Read the model definition and answer for the solid it produces. Units are mm, in the model's axes. Coordinates: 2 decimals unless noted, no trailing zeros. Order: outer loops, then holes, each group sorted by start corner. A loop starts at its lowest first (then second) coordinate and runs counter-clockwise, first axis right, second up. Notation, with made-up numbers: M 55,73.5 L 60,73.5 A14 cw 60,97.5 Z; hole C -32,27.5 d5. An arc over 180 degrees is marked long. Write each question's results on one line, items separated by ' | '.
Autodesk Inventor part; units mm, degrees
ref_plane "YZ Plane" through (0, 0, 0) normal (1, 0, 0) x (0, 1, 0)
ref_plane "XZ Plane" through (0, 0, 0) normal (0, 1, 0) x (-1, 0, 0)
ref_plane "XY Plane" through (0, 0, 0) normal (0, 0, 1) x (1, 0, 0)
sketch "Sketch1" plane through (0, 0, 0) normal (0, 1, 0) x (-1, 0, 0)
  line L0 (0, 0) -> (-95, 0)
  line L1 (-95, 0) -> (-95, -95)
  line L2 (-95, -95) -> (0, -95)
  line L3 (0, -95) -> (0, 0)
  line L4 (0, 0) -> (-5, 0)
  line L5 (-5, 0) -> (-5, -5)
  line L6 (-5, -5) -> (0, -5)
  line L7 (0, -5) -> (0, 0)
  line L8 (-95, -95) -> (-90, -95)
  line L9 (-90, -95) -> (-90, -90)
  line L10 (-90, -90) -> (-95, -90)
  line L11 (-95, -90) -> (-95, -95)
  line L12 (-90, -90) -> (-5, -90)
  line L13 (-5, -90) -> (-5, -5)
  line L14 (-5, -5) -> (-90, -5)
  line L15 (-90, -5) -> (-90, -90)
  line L16 (0, -47.5) -> (0, 0)
  line L17 (0, -47.5) -> (0, -95)
  line L18 (0, -23.75) -> (0, -18.75)
  line L19 (0, -18.75) -> (0, -28.75)
  line L20 (0, -71.25) -> (0, -76.25)
  line L21 (0, -76.25) -> (0, -66.25)
  line L22 (0, -18.75) -> (0, -28.75) construction
  line L23 (-5, -18.75) -> (-5, -28.75)
  line L24 (5, -28.75) -> (5, -18.75)
  arc A0 (5, -18.75) -> (-5, -18.75) centre (0, -18.75) ccw
  arc A1 (-5, -28.75) -> (5, -28.75) centre (0, -28.75) ccw
  line L25 (0, -66.25) -> (0, -76.25) construction
  line L26 (-5, -66.25) -> (-5, -76.25)
  line L27 (5, -76.25) -> (5, -66.25)
  arc A2 (5, -66.25) -> (-5, -66.25) centre (0, -66.25) ccw
  arc A3 (-5, -76.25) -> (5, -76.25) centre (0, -76.25) ccw
  point P0 (0, -61.25)
  point P1 (0, -81.25)
  point P2 (0, -13.75)
  point P3 (0, -33.75)
  dimension "d0" = 95
  dimension "d1" = 95
  dimension "d2" = 5
  dimension "d3" = 5
  dimension "d4" = 5
  dimension "d5" = 5
  dimension "d8" = 5
  dimension "d9" = 10
  dimension "d10" = 5
  dimension "d11" = 10
  dimension "d12" = 10
  dimension "d13" = 10
extrude "Extrusion1" add sketch "Sketch1" along normal blind 1.5 contours L3 L6 L5 L0 | L5 L14 L15 L10 L1 L0 | L3 A0 L13 L6 | A0 L24 A1 L3 | L3 A1 L13 A0 | L10 L9 L2 L1 | L12 L13 A3 L3 L2 L9 | A1 L3 A2 L13 | A2 L3 A3 L13 | A2 L27 A3 L3
fillet "Fillet1" radius 8 8 edges at (5, 0.75, -5) (0, 0.75, 0) (0, 0.75, -95) (5, 0.75, -90) (95, 0.75, 0) (90, 0.75, -5) (95, 0.75, -95) (90, 0.75, -90)
fillet "Fillet2" radius 1 12 edges at (-3.5355, 0, -15.2145) (-3.5355, 0, -32.2855) (-5, 0, -23.75) (-3.5355, 1.5, -15.2145) (-3.5355, 1.5, -32.2855) (-5, 1.5, -23.75) (-3.5355, 0, -62.7145) (-3.5355, 0, -79.7855) (-5, 0, -71.25) (-3.5355, 1.5, -62.7145) (-3.5355, 1.5, -79.7855) (-5, 1.5, -71.25)
properties part number "Plate"
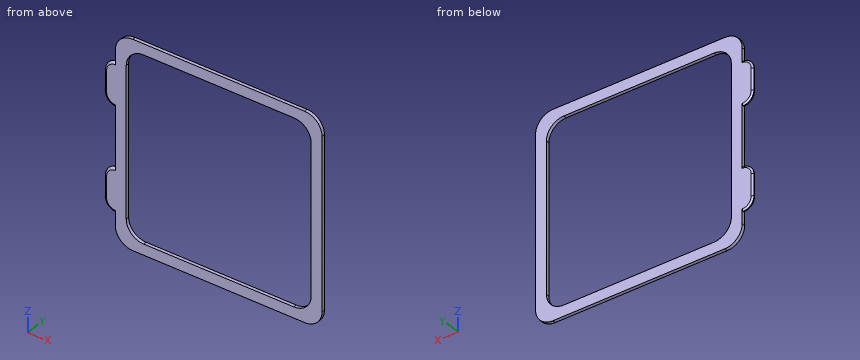
(1) The part is cut by section A-A, the plane z = -43.5. Write down the section's boundary in (x, y), then the cut area to 3 significant figures.
Conclusion:
outline: M 0,0 L 5,0 L 5,1.5 L 0,1.5 Z; M 90,0 L 95,0 L 95,1.5 L 90,1.5 Z | area: 15.0 mm²
(2) Straight lines are drawn through the part: line 1 (X direction, y = 1.05, z = -13); line 2 (Z direction, x = 62, y = 0.7); line 3 (X direction, y = 0.4, z = -66). For each, find the intervals that lie inside material, in ascending order.
Conclusion:
line 1: 0 to 5, 90 to 95 | line 2: -95 to -90, -5 to 0 | line 3: -4.79 to 5, 90 to 95
(3) The part is cut by section C-C, the plane z = -68.5. Write down the section's boundary in (x, y).
Conclusion:
outline: M -5,1 A1 ccw -4,0 L 5,0 L 5,1.5 L -4.13,1.5 A1 ccw Z; M 90,0 L 95,0 L 95,1.5 L 90,1.5 Z
(4) The part is cut by section D-D, the plane y = 0.6. Write down the section's boundary in (x, z).
Conclusion:
outline: M -4.92,-76.25 A4.92 ccw 0,-81.17 L 0,-87 A8 ccw 8,-95 L 87,-95 A8 ccw 95,-87 L 95,-8 A8 ccw 87,0 L 8,0 A8 ccw 0,-8 L 0,-13.83 A4.92 ccw -4.92,-18.75 L -4.92,-28.75 A4.92 ccw 0,-33.67 L 0,-61.33 A4.92 ccw -4.92,-66.25 Z; hole M 5,-82 A8 ccw 13,-90 L 82,-90 A8 ccw 90,-82 L 90,-13 A8 ccw 82,-5 L 13,-5 A8 ccw 5,-13 Z
(5) Given pin 1 (0.8 mm diameter, centred on x = 43.5, y = 0.5, fed in from +Z), flat-ended and moving along its own axis, determine where the tip first touches the part or whether it passes through.
Conclusion:
pin 1: z = 0
(6) The part is cut by section B-B, the plane x = 21.5. Write down the section's boundary in (y, z), then the cut area to 3 significant figures.
Conclusion:
outline: M 0,-95 L 1.5,-95 L 1.5,-90 L 0,-90 Z; M 0,-5 L 1.5,-5 L 1.5,0 L 0,0 Z | area: 15.0 mm²
